Design review of the part built by this model. Coordinates are the model's own, in mm. Face numbers are marked on the shaded views. A direction names the side the tool comes from. Give positions to 0.01 mm unless a question says otherwise; leave off trailing zeros. Order: outer loops, then holes, each group sorted by start corner. A loop starts at its lowest first (then second) coordinate and runs counter-clockwise, first axis right, second up. Notation, with made-up numbers: (-20, 54.5) -> (8, 54.5) arc R34 ccw to (8, 87.5) -> close; hole circle Ø8 at (35.25, 29). An arc over 180 degrees is marked (long way). One line per item, written item: value.
from build123d import *

# Parameters (mm, degrees)
F3_R     = 78.8340785065
F4_DEPTH = 40
F6_DEPTH = 5
F7_R     = 4.99999


# Not quite as in the source:
# - a fillet or chamfer that OpenCascade refuses, or shapes differently, is made with other operations: its cross-section is extruded or revolved along the edge and cut away or added
# - a fillet or chamfer is up to 0.001 mm smaller than in the source, because OpenCascade refuses the exact size
# - ends of sketch curves that miss each other by under 0.0002 mm in the source are joined
# - a feature names something its author has since deleted; it is built from what else it names


with BuildPart() as f1:
    # F0 (on Top) → F1 (revolve)
    with BuildSketch(Plane.XY):
        with BuildLine():
            Line((0, -49), (0, -9))
            Line((0, -9), (-31, -9))
            Line((-31, -9), (-31, -6.5))
            Line((-31, -6.5), (-36, -6.5))
            Line((-36, -6.5), (-36, -11.5))
            Line((-36, -11.5), (-57.0000335574, -11.5))
            Line((-57.0000335574, -11.5), (-57.0000000106, -49))
            Line((-57.0000000106, -49), (-54.0000000106, -49))
            Line((-54.0000000106, -49), (-54.0000000106, -44.8544277911))
            ThreePointArc((-54.0000000106, -44.8544277911), (-47.2635467929, -28.5904424478), (-31, -21.8529305247))
            Line((-31, -21.8529305247), (-26.0000000106, -21.8529305247))
            ThreePointArc((-26.0000000106, -21.8529305247), (-9.7364532177, -28.5904424478), (-3, -44.8544277911))
            Line((-3, -44.8544277911), (-3, -49))
            Line((-3, -49), (0, -49))
        make_face()
    revolve(axis=Axis((7.519562263, 0, 0), (1, 0, 0)))

    # F2: fillet of radius 5 on 1 edges, made by hand

    # F2_s1 → F2_t2 (revolve, cut)
    with BuildSketch(Plane.XY):
        with BuildLine():
            ThreePointArc((-3.0028205283, -44.4942267471), (-2.1641233212, -47.188770834), (0, -49))
            Line((0, -49), (-0.1996566353, -49.458407273))
            ThreePointArc((-0.1996566353, -49.458407273), (-1.5, -49.5), (-3, -49.5))
            Line((-3, -49.5), (-3.5, -49))
            ThreePointArc((-3.5, -49), (-3.5, -44.8544277911), (-3.5027592164, -44.5020566949))
            Line((-3.5027592164, -44.5020566949), (-3.0028205283, -44.4942267471))
        make_face()
    revolve(axis=Axis((-3, 0, 0), (1, 0, 0)), mode=Mode.SUBTRACT)

    # F3 (on face) → F4 (cut)
    with BuildSketch(Plane.YZ.offset(-31)):
        Circle(F3_R)
    extrude(amount=F4_DEPTH, mode=Mode.SUBTRACT)

    # F5 (on face) → F6 (join)
    with BuildSketch(Plane.YZ.offset(-31)):
        with BuildLine():
            Line((9, 0), (21.85, 0))
            ThreePointArc((21.85, 0), (20.1867677854, 8.3616329972), (15.4502831689, 15.4502831689))
            Line((15.4502831689, 15.4502831689), (6.3639610307, 6.3639610307))
            ThreePointArc((6.3639610307, 6.3639610307), (8.3149157926, 3.4441508913), (9, 0))
        make_face()
        with BuildLine():
            Line((0, 9), (0, 21.85))
            ThreePointArc((0, 21.85), (-8.3616329972, 20.1867677854), (-15.4502831689, 15.4502831689))
            Line((-15.4502831689, 15.4502831689), (-6.3639610307, 6.3639610307))
            ThreePointArc((-6.3639610307, 6.3639610307), (-3.4441508913, 8.3149157926), (0, 9))
        make_face()
        with BuildLine():
            ThreePointArc((0, -21.85), (8.3616329972, -20.1867677854), (15.4502831689, -15.4502831689))
            Line((15.4502831689, -15.4502831689), (6.3639610307, -6.3639610307))
            ThreePointArc((6.3639610307, -6.3639610307), (3.4441508913, -8.3149157926), (0, -9))
            Line((0, -9), (0, -21.85))
        make_face()
        with BuildLine():
            ThreePointArc((-21.85, 0), (-20.1867677854, -8.3616329972), (-15.4502831689, -15.4502831689))
            Line((-15.4502831689, -15.4502831689), (-6.3639610307, -6.3639610307))
            ThreePointArc((-6.3639610307, -6.3639610307), (-8.3149157926, -3.4441508913), (-9, 0))
            Line((-9, 0), (-21.85, 0))
        make_face()
    extrude(amount=F6_DEPTH)

    # F7 (radius 5 in the source; OpenCascade refuses exactly that, so slightly less here)
    f7_edges = [f1.edges().sort_by_distance(p)[0] for p in [
        (-36, 11.5, 0),
    ]]
    fillet(f7_edges, radius=F7_R)


solid = f1.part
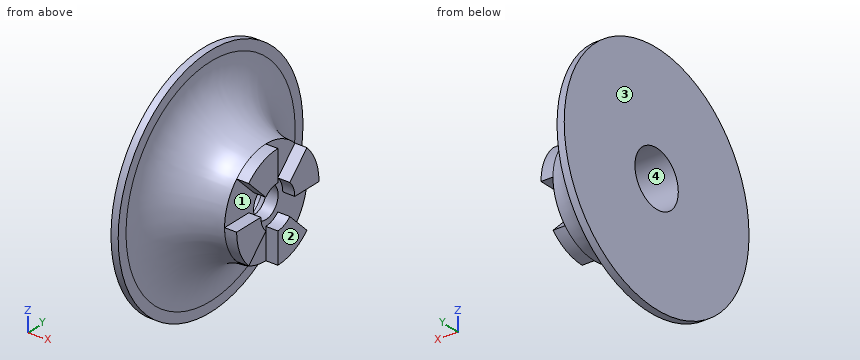
Item 1: To check wall thickness, follow line 1 along Y through (x, z) = (-32, 0); line 2 along Z through (x, y) = (-33.45, 0); line 3 along Z through (x, y) = (-34.35, 0). State the ranges of each line that lie inside material, in increasing order. Write a range as from..to.
Returned:
line 1: -21.87..-6.5, 6.5..21.87
line 2: -21.98..-6.5, 6.5..21.98
line 3: -22.1..-6.5, 6.5..22.1
Item 2: Draft analysis for pull direction Z (two halves, no side actions). For the marked faces 1 and 2, state which applies: pulls with the +Z half, pulls with the -Z half, needs draft (parallel to the pull), parting line crosses it, or undercut.
Returned:
face 1: undercut
face 2: needs draft
Item 3: Add section B-B on x = -49.5. Give the boundary of the cut face in (y, z), plus the area to 3 significant figures.
Returned:
outline: circle Ø62.38 at (0, 0); hole circle Ø23 at (0, 0)
area: 2,640 mm²
Item 4: Clearance check with flat-ended pins moving along their axes: P1, Ø4, axis at x = -28, z = -15.5, coming from the -Y side; P2, Ø1, axis at x = -50.5, y = 38.5, coming from the +Z side (3 decimals); P3, Ø10, axis at x = -40.5, z = -24, coming from the +Y side; P4, Ø4, axis at x = -28.5, y = -12.5, coming from the +Z side. State where each tip first meets the part, or that it passes through.
Returned:
P1: y = -17.18
P2: through
P3: y = 15.91
P4: z = 19.16
Item 5: Machinability: for the marked faces 3 and 4, which of the approach directions +Z, -Z, +X, -X, +Y, -Y give a long, thin tool a straight path to every point of the face, cutting with its end or side? Answer none if there is none.
Returned:
face 3: +Z, -Z, -X, +Y, -Y
face 4: -X
Item 6: Add section A-A on x = -44.5. Give the boundary of the cut face in (y, z).
Returned:
outline: circle Ø52.46 at (0, 0); hole circle Ø23 at (0, 0)
